```python
from build123d import *

# Parameters (mm, degrees)
F0_R     = 2.0193
F0_R_2   = 14.2875
F0_R_3   = 2.5527
F0_R_4   = 2.8575
F1_DEPTH = 6.35
F3_DEPTH = 6.351
F4_R     = 6.35


with BuildPart() as f1:
    # F0 (on Front) → F1 (new body)
    with BuildSketch(Plane.XZ):
        with BuildLine():
            ThreePointArc((-48.749763, 42.283305), (-62.529838, 29.799935), (-80.924107, 27.084083))
            ThreePointArc((-80.924107, 27.084083), (-84.247136, 25.334263), (-83.576453, 21.639053))
            Line((-83.576453, 21.639053), (-42.467369, -17.309619))
            ThreePointArc((-42.467369, -17.309619), (-40.450683, -18.59888), (-38.1, -19.05))
            Line((-38.1, -19.05), (38.1, -19.05))
            ThreePointArc((38.1, -19.05), (40.450683, -18.59888), (42.467369, -17.309619))
            Line((42.467369, -17.309619), (83.576453, 21.639053))
            ThreePointArc((83.576453, 21.639053), (84.247136, 25.334263), (80.924107, 27.084083))
            ThreePointArc((80.924107, 27.084083), (62.529838, 29.799935), (48.749763, 42.283305))
            Line((48.749763, 42.283305), (23.147521, 84.995065))
            ThreePointArc((23.147521, 84.995065), (0, 98.1075), (-23.147521, 84.995065))
            Line((-23.147521, 84.995065), (-48.749763, 42.283305))
        make_face()
        with Locations((-38.1, -12.7)):
            Circle(F0_R, mode=Mode.SUBTRACT)
        with Locations((-38.1, 0)):
            Circle(F0_R, mode=Mode.SUBTRACT)
        Circle(F0_R_2, mode=Mode.SUBTRACT)
        with Locations((-38.1, 12.7)):
            Circle(F0_R, mode=Mode.SUBTRACT)
        with Locations((38.1, -12.7)):
            Circle(F0_R, mode=Mode.SUBTRACT)
        with Locations((38.1, 0)):
            Circle(F0_R, mode=Mode.SUBTRACT)
        with Locations((38.1, 12.7)):
            Circle(F0_R, mode=Mode.SUBTRACT)
        with Locations((-41.275, 40.64)):
            Circle(F0_R_3, mode=Mode.SUBTRACT)
        with Locations((-25.4, 71.12)):
            Circle(F0_R_4, mode=Mode.SUBTRACT)
        with Locations((0, 71.12)):
            Circle(F0_R_2, mode=Mode.SUBTRACT)
        with Locations((41.275, 40.64)):
            Circle(F0_R_3, mode=Mode.SUBTRACT)
        with Locations((25.4, 71.12)):
            Circle(F0_R_4, mode=Mode.SUBTRACT)
    extrude(amount=F1_DEPTH)

    # F2 (on face) → F3 (cut, through all)
    with BuildSketch(Plane.XZ.offset(6.35)):
        with BuildLine():
            Line((3.96875, 49.252224), (3.96875, 21.867776))
            ThreePointArc((3.96875, 21.867776), (11.982359, 18.718272), (18.19753, 12.759331))
            Line((18.19753, 12.759331), (32.248092, 17.442852))
            Line((32.248092, 17.442852), (34.551338, 37.71141))
            Line((34.551338, 37.71141), (13.361087, 53.359595))
            ThreePointArc((13.361087, 53.359595), (8.904967, 50.75699), (3.96875, 49.252224))
        make_face()
        with BuildLine():
            ThreePointArc((-18.19753, 12.759331), (-11.982359, 18.718272), (-3.96875, 21.867776))
            Line((-3.96875, 21.867776), (-3.96875, 49.252224))
            ThreePointArc((-3.96875, 49.252224), (-8.904967, 50.75699), (-13.361087, 53.359595))
            Line((-13.361087, 53.359595), (-34.551338, 37.71141))
            Line((-34.551338, 37.71141), (-32.248092, 17.442852))
            Line((-32.248092, 17.442852), (-18.19753, 12.759331))
        make_face()
    extrude(amount=-F3_DEPTH, mode=Mode.SUBTRACT)

    # F4
    f4_edges = [f1.edges().sort_by_distance(p)[0] for p in [
        (-13.361087, -3.175, 53.359595),
        (-3.96875, -3.175, 49.252224),
        (-3.96875, -3.175, 21.867776),
        (-18.19753, -3.175, 12.759331),
        (-32.248092, -3.175, 17.442852),
        (-34.551338, -3.175, 37.71141),
        (3.96875, -3.175, 49.252224),
        (13.361087, -3.175, 53.359595),
        (34.551338, -3.175, 37.71141),
        (32.248092, -3.175, 17.442852),
        (18.19753, -3.175, 12.759331),
        (3.96875, -3.175, 21.867776),
    ]]
    fillet(f4_edges, radius=F4_R)


solid = f1.part
```
Check sheet for the modelled part. Datum: model origin and axes. Units: mm. A direction names the side the tool comes from. Round coordinates to 2 decimals unless told otherwise and drop trailing zeros. Loops run counter-clockwise (first coordinate to the right, second up) from the corner with the lowest first, then second, coordinate; pieces in that order, holes last. Notation, with made-up numbers: (21.5, 62.5) - (57.5, 62.5) arc R24 ccw to (57.5, 73.5) - close; hole circle Ø3 at (45.25, 71). An arc over 180 degrees is marked (long way). Write item = value, one per line. Start each with the question number.
Q1. Access from +Z, -Z, +X, -X, +Y, -Y to the whole of each face (thin tool, end or side, straight path). Record for faces 4 (the face through (36.13, -3.13, 63.34)), 5 (the face through (33.668, -3.131, 37.276)).
Q2. Release check for a two-part mould opening along Z. For faces 1 (the face through (-63.31, -3.13, 2.44)), 2 (the face through (-1, 0, 27)), 3 (the face through (31.3, -3.13, 18.15)) record: pulls with the +Z half, pulls with the -Z half, needs draft (parallel to the pull), parting line crosses it, or undercut.
Q3. Section check A-A (x = 0). Record the boundary of the cut face in (y, z), plus the area to 3 significant figures.
Q4. Section check D-D (x = 25.4). Record the boundary of the cut face in (y, z), plus the area to 3 significant figures.
Q5. Section check B-B (z = 60). Record the boundary of the cut face in (x, y).
Q6. Section check C-C (y = -4). Count the separate pieces of the cut face and the enclosed holes in it, plus the area to 3 significant figures.
Q7. Thickness scan on L1, parallel to Z at x = 1, y = -1.25; L2, parallel to Z at x = 0, y = -1.5; L3, parallel to Z at x = -38.1, y = -4.75. Record the ranges inside material, lowest first.
Q8. Depth check by flat-ended pin: P1, Ø3, axis at x = 61.5, y = -5, coming from the +Z side; P2, Ø2, axis at y = -1.5, z = 13, coming from the -X side; P3, Ø3, axis at y = -2, z = 86, coming from the -X side. Enter the tip coordinate at first touch or a pass-through.
Derived:
q1.face_4 = +Z, +X, +Y, -Y
q1.face_5 = +Y, -Y
q2.face_1 = pulls with the -Z half
q2.face_2 = needs draft
q2.face_3 = undercut
q3.outline = (-6.35, -19.05) - (0, -19.05) - (0, -14.29) - (-6.35, -14.29) - close; (-6.35, 14.29) - (0, 14.29) - (0, 56.83) - (-6.35, 56.83) - close; (-6.35, 85.41) - (0, 85.41) - (0, 98.11) - (-6.35, 98.11) - close
q3.area = 381 mm^2
q4.outline = (-6.35, -19.05) - (0, -19.05) - (0, 15.16) - (-6.35, 15.16) - close; (-6.35, 44.47) - (0, 44.47) - (0, 68.26) - (-6.35, 68.26) - close; (-6.35, 73.98) - (0, 73.98) - (0, 81.24) - (-6.35, 81.24) - close
q4.area = 414 mm^2
q5.outline = (-38.13, -6.35) - (-8.97, -6.35) - (-8.97, 0) - (-38.13, 0) - close; (8.97, -6.35) - (38.13, -6.35) - (38.13, 0) - (8.97, 0) - close
q6.separate_pieces = 1
q6.enclosed_holes = 14
q6.area = 7,960 mm^2
q7.L1 = -19.05 to -14.25, 14.25 to 56.87, 85.37 to 98.09
q7.L2 = -19.05 to -14.29, 14.29 to 56.83, 85.41 to 98.11
q7.L3 = -19.05 to -14.72, -10.68 to -2.02, 2.02 to 10.68, 14.72 to 60.05
q8.P1 = 31.14
q8.P2 = -75.51
q8.P3 = -23.44
